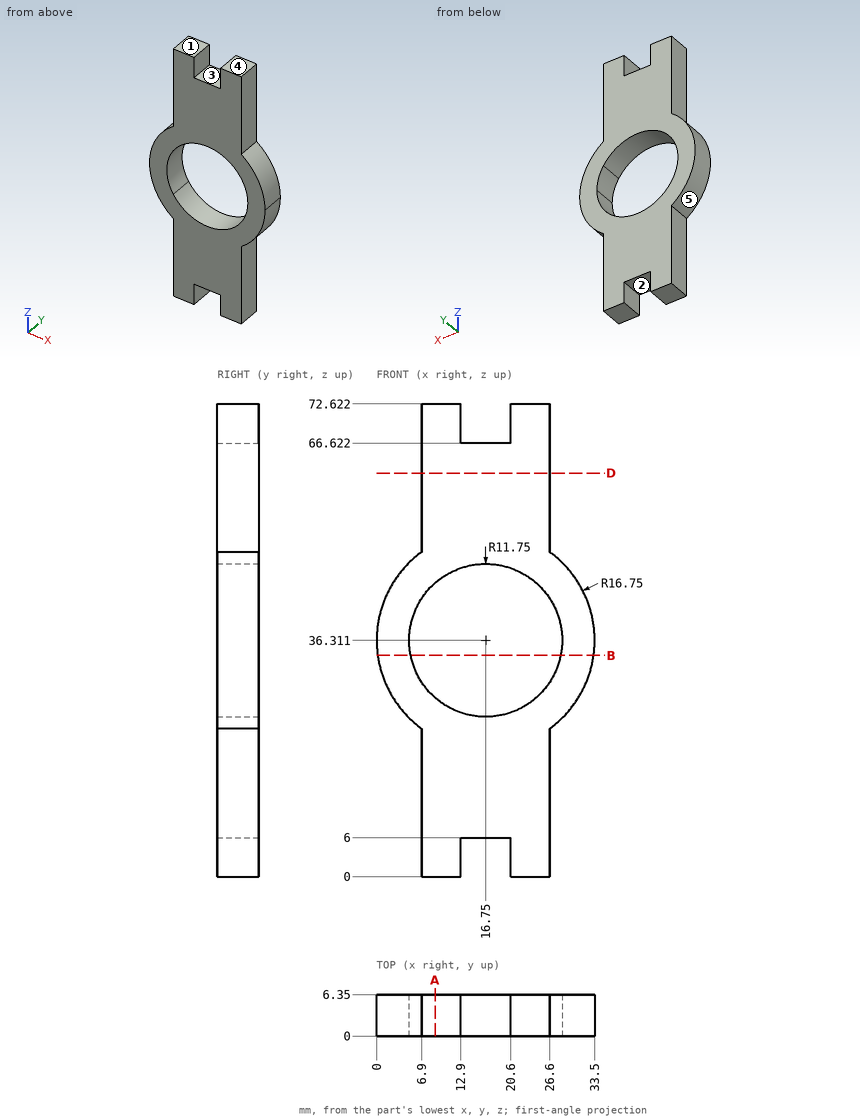
Check sheet for the drawn part. Datum: minimum x, y, z corner. Units: mm. A direction names the side the tool comes from. Coordinates: 2 decimals unless noted, no trailing zeros. Loops run counter-clockwise (first coordinate to the right, second up) from the corner with the lowest first, then second, coordinate; pieces in that order, holes last. Notation, with made-up numbers: (14.25, -9.5) -> (73.25, -9.5) arc R37 cw to (73.25, 29.5) -> close; hole circle Ø10 at (-28, -1.75). An arc over 180 degrees is marked (long way). Answer in a Markdown table with one row per item.
1. Sectioned sample at B-B, the plane z = 34. Record the boundary of the cut face in (x, y), then the cut area to 3 significant figures.
Check values:
| item | result |
|---|---|
| outline | (0.16, 0) -> (5.23, 0) -> (5.23, 6.35) -> (0.16, 6.35) -> close; (28.27, 0) -> (33.34, 0) -> (33.34, 6.35) -> (28.27, 6.35) -> close |
| area | 64.4 mm2 |
2. Go/stop test with flat-tipped pins: pin 1 (1.9 mm diameter, centred on x = 16.5, y = 4, fed in from +Z); pin 2 (3 mm diameter, centred on y = 5.5, z = 43.5, fed in from -X); pin 3 (3 mm diameter, centred on y = 3.5, z = 57.5, fed in from +X). Record where each tip stops, or that it passes through.
Check values:
| item | result |
|---|---|
| pin 1 | stops at z = 66.62 |
| pin 2 | stops at x = 1 |
| pin 3 | stops at x = 26.6 |
3. Sectioned sample at D-D, the plane z = 62. Record the boundary of the cut face in (x, y), then the cut area to 3 significant figures.
Check values:
| item | result |
|---|---|
| outline | (6.9, 0) -> (26.6, 0) -> (26.6, 6.35) -> (6.9, 6.35) -> close |
| area | 125 mm2 |
4. Access from +Z, -Z, +X, -X, +Y, -Y to the whole of each face (thin tool, end or side, straight path). Record for the marked faces 1 and 2.
Check values:
| item | result |
|---|---|
| face 1 | +Z, +X, -X, +Y, -Y |
| face 2 | -Z, +Y, -Y |
5. Release check for a two-part mould opening along X. For the marked faces 3, 4 and 5 record: released by +X, released by -X, zero draft, split by the parting line, or undercut.
Check values:
| item | result |
|---|---|
| face 3 | undercut |
| face 4 | zero draft |
| face 5 | released by -X |
6. Sectioned sample at A-A, the plane x = 9. Record the boundary of the cut face in (y, z), then the cut area to 3 significant figures.
Check values:
| item | result |
|---|---|
| outline | (0, 0) -> (6.35, 0) -> (6.35, 27.48) -> (0, 27.48) -> close; (0, 45.14) -> (6.35, 45.14) -> (6.35, 72.62) -> (0, 72.62) -> close |
| area | 349 mm2 |
7. Material ranges on line 1 along X through (y, z) = (5, 67.5); line 2 along Z through (x, y) = (16.5, 3); line 3 along X through (y, z) = (4, 52), recorded low to high. Write a range as [from, to].
Check values:
| item | result |
|---|---|
| line 1 | x = [6.9, 12.9], [20.6, 26.6] |
| line 2 | z = [6, 24.56], [48.06, 66.62] |
| line 3 | x = [6.9, 26.6] |
